from build123d import *

# Parameters (mm, degrees)
F0_W     = 43.9917519689
F0_H     = 8.7983510457
F1_DEPTH = 25.4
F3_DEPTH = 25.4


with BuildPart() as f1:
    # F0 (on Front) → F1 (new body)
    with BuildSketch(Plane.XZ):
        with Locations((3.4826807678, 0.0916493591)):
            Rectangle(F0_W, F0_H)
    extrude(amount=F1_DEPTH)

    # F2 (on face) → F3 (join)
    with BuildSketch(Plane.XZ.offset(25.4)):
        Polygon((-7.7598788776, 11.3449869677), (-12.6920454204, 4.4908248819), (22.3263110965, 4.4908248819), (17.1475466341, 11.3449869677), align=None)
    extrude(amount=-F3_DEPTH)


solid = f1.part
The listing builds one solid part. Answer for the finished solid, in the listing's coordinates (mm). A direction names the side the tool comes from. Round coordinates to 2 decimals unless told otherwise and drop trailing zeros. Order: outer loops, then holes, each group sorted by start corner. A loop starts at its lowest first (then second) coordinate and runs counter-clockwise, first axis right, second up. Notation, with made-up numbers: (84.25, 66) -> (96.25, 66) arc R28 cw to (96.25, 96) -> close; hole circle Ø11 at (62.25, 60.5). An arc over 180 degrees is marked (long way). Write each question's results on one line, items separated by ' | '. Start each with the question number.
Q1. Find section C-C (z = 6.5). Determine the outline of the cut face in (x, y), then the cut area to 3 significant figures.
Q2. Find section B-B (x = -14.5). Determine the outline of the cut face in (y, z), then the cut area to 3 significant figures.
Q3. Straight lines are drawn through the part: probe 1 along Z at (x, y) = (-13, -18.75); probe 2 along X at (y, z) = (-24, 10); probe 3 along Z at (x, y) = (-9.5, -13.5). For each, find the intervals that lie inside material, in ascending order. Write a range as from..to.
Q4. Which of the six approach directions +Z, -Z, +X, -X, +Y, -Y give full straight-line access (tool end or side, diameter ignored) to faces 1 (the flat face through (-16, -13, 4.491)), 2 (the flat face through (25.479, -13, 0)), 3 (the flat face through (24, -13, 4.491))?
Q5. Each of these flat-tipped pins is pushed along its axis until it touches: pin 1 (0.9 mm diameter, centred on x = 24.5, y = -17.5, fed in from +Z); pin 2 (1.5 mm diameter, centred on y = -12, z = 8.5, fed in from +X). Where does it stop, or does it pass through?
Q6. Find section A-A (y = -11). Determine the outline of the cut face in (x, z), then the cut area to 3 significant figures.
Worked answers:
1) outline: (-11.25, -25.4) -> (20.81, -25.4) -> (20.81, 0) -> (-11.25, 0) -> close | area: 814 mm2
2) outline: (-25.4, -4.31) -> (0, -4.31) -> (0, 4.49) -> (-25.4, 4.49) -> close | area: 223 mm2
3) probe 1: z = -4.31..4.49 | probe 2: x = -8.73..18.16 | probe 3: z = -4.31..8.93
4) face 1: +Z, -X, +Y, -Y | face 2: +Z, -Z, +X, +Y, -Y | face 3: +Z, +X, +Y, -Y
5) pin 1: stops at z = 4.49 | pin 2: stops at x = 19.86
6) outline: (-18.51, -4.31) -> (25.48, -4.31) -> (25.48, 4.49) -> (22.33, 4.49) -> (17.15, 11.34) -> (-7.76, 11.34) -> (-12.69, 4.49) -> (-18.51, 4.49) -> close | area: 592 mm2
